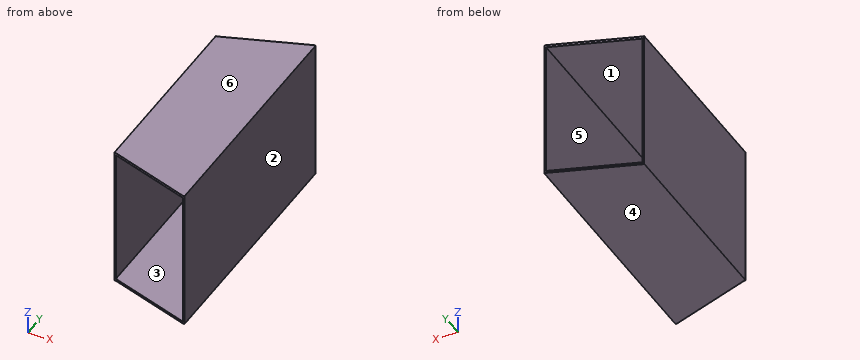
```python
from build123d import *

# Parameters (mm, degrees)
SKETCH1_W           = 15
SKETCH1_H           = 44.271951098
BOSS_EXTRUDE4_DEPTH = 25
SKETCH4_W           = 14.437791502
SKETCH4_H           = 24.200488612
CUT_EXTRUDE4_DEPTH  = 54.009486453
CUT_EXTRUDE5_DEPTH  = 54.009486453
CUT_EXTRUDE6_DEPTH  = 54.009486453
SKETCH7_W           = 0.258481213
SKETCH7_H           = 5
CUT_EXTRUDE7_DEPTH  = 54.009486453
SKETCH10_W          = 0.258481213
SKETCH10_H          = 5
CUT_EXTRUDE8_DEPTH  = 54.009486453


with BuildPart() as part:
    # Sketch1 → Boss-Extrude4 (new body)
    with BuildSketch(Plane.XY):
        with Locations((7.5, 22.135975549)):
            Rectangle(SKETCH1_W, SKETCH1_H)
    extrude(amount=BOSS_EXTRUDE4_DEPTH)

    # Sketch4 → Cut-Extrude4 (cut, through all)
    with BuildSketch(Plane(origin=(0, 44.271951098, 0), x_dir=(1, 0, 0), z_dir=(0, 1, 0))):
        with Locations((7.477376964, -12.479096566)):
            Rectangle(SKETCH4_W, SKETCH4_H)
    extrude(amount=-CUT_EXTRUDE4_DEPTH, mode=Mode.SUBTRACT)

    # Sketch5 → Cut-Extrude5 (cut, through all)
    with BuildSketch(Plane(origin=(0, 0, 0), x_dir=(-1, 0, 0), z_dir=(0, 0, -1))):
        Polygon((-14.696272715, 44.271951098), (-0.258481213, 44.271951098), (-0.258481213, 39.271951098), align=None)
    extrude(amount=-CUT_EXTRUDE5_DEPTH, mode=Mode.SUBTRACT)

    # Sketch6 → Cut-Extrude6 (cut, through all)
    with BuildSketch(Plane(origin=(0, 0, 0), x_dir=(-1, 0, 0), z_dir=(0, 0, -1))):
        Polygon((-0.258481213, 0), (-0.258481213, 5), (-14.696272715, 0), align=None)
    extrude(amount=-CUT_EXTRUDE6_DEPTH, mode=Mode.SUBTRACT)

    # Sketch7 → Cut-Extrude7 (cut, through all)
    with BuildSketch(Plane(origin=(0, 0, 0), x_dir=(-1, 0, 0), z_dir=(0, 0, -1))):
        with Locations((-0.129240607, 41.771951098)):
            Rectangle(SKETCH7_W, SKETCH7_H)
    extrude(amount=-CUT_EXTRUDE7_DEPTH, mode=Mode.SUBTRACT)

    # Sketch10 → Cut-Extrude8 (cut, through all)
    with BuildSketch(Plane(origin=(0, 0, 0), x_dir=(-1, 0, 0), z_dir=(0, 0, -1))):
        with Locations((-0.129240607, 2.5)):
            Rectangle(SKETCH10_W, SKETCH10_H)
    extrude(amount=-CUT_EXTRUDE8_DEPTH, mode=Mode.SUBTRACT)


solid = part.part
```
Can you work these out from the model? Positions are in its coordinate system, mm. Face numbers are marked on the shaded views. A direction names the side the tool comes from. Give positions to 0.01 mm unless a question says otherwise; leave off trailing zeros. Loops run counter-clockwise (first coordinate to the right, second up) from the corner with the lowest first, then second, coordinate; pieces in that order, holes last. Notation, with made-up numbers: M 85.25,87.25 L 123.25,87.25 A20 ccw 123.25,113.25 Z; hole C 58.5,-29 d1. An arc over 180 degrees is marked long. Answer in a Markdown table with one row per item.
1. Suppose I cut it at C-C on x = 3.75. Write out the boundary of the cut face in (y, z).
Taken from the geometry:
| item | result |
|---|---|
| outline | M 3.79,0 L 40.48,0 L 40.48,0.38 L 3.79,0.38 Z; M 3.79,24.58 L 40.48,24.58 L 40.48,25 L 3.79,25 Z |
2. Thinking about a two-plate mould opening in X: for the marked faces 1, 2, 3 and 4, which applies, released by +X, released by -X, zero draft, split by the parting line, or undercut?
Taken from the geometry:
| item | result |
|---|---|
| face 1 | undercut |
| face 2 | released by +X |
| face 3 | undercut |
| face 4 | zero draft |
3. Which directions (+Z, -Z, +X, -X, +Y, -Y) give clear straight access to the entire face, cutting with the end or side of a thin tool? Please do the marked faces 5 and 6.
Taken from the geometry:
| item | result |
|---|---|
| face 5 | +Y, -Y |
| face 6 | +Z, +X, -X, +Y, -Y |
4. If I drill on line 1 along X through (y, z) = (26, 10.5); line 2 along Z through (x, y) = (10, 5.5); line 3 along X through (y, z) = (42.5, 5.5), over which ranges is the centre line in solid material (lowest first)?
Taken from the geometry:
| item | result |
|---|---|
| line 1 | x = 0 to 0.26, 14.7 to 15 |
| line 2 | z = 0 to 0.38, 24.58 to 25 |
| line 3 | x = 14.7 to 15 |
5. Suppose I cut it at D-D on y = 4.5. Write out the boundary of the cut face in (x, z), plus the area to 3 significant figures.
Taken from the geometry:
| item | result |
|---|---|
| outline | M 1.7,0 L 15,0 L 15,25 L 1.7,25 L 1.7,24.58 L 14.7,24.58 L 14.7,0.38 L 1.7,0.38 Z |
| area | 18.0 mm² |
6. Suppose I cut it at A-A on y = 31. Write out the boundary of the cut face in (x, z), plus the area to 3 significant figures.
Taken from the geometry:
| item | result |
|---|---|
| outline | M 0,0 L 15,0 L 15,25 L 0,25 Z; hole M 0.26,0.38 L 14.7,0.38 L 14.7,24.58 L 0.26,24.58 Z |
| area | 25.6 mm² |
7. Suppose I cut it at B-B on z = 15. Write out the boundary of the cut face in (x, y), plus the area to 3 significant figures.
Taken from the geometry:
| item | result |
|---|---|
| outline | M 0,5 L 0.26,5 L 0.26,39.27 L 0,39.27 Z; M 14.7,0 L 15,0 L 15,44.27 L 14.7,44.27 Z |
| area | 22.3 mm² |
